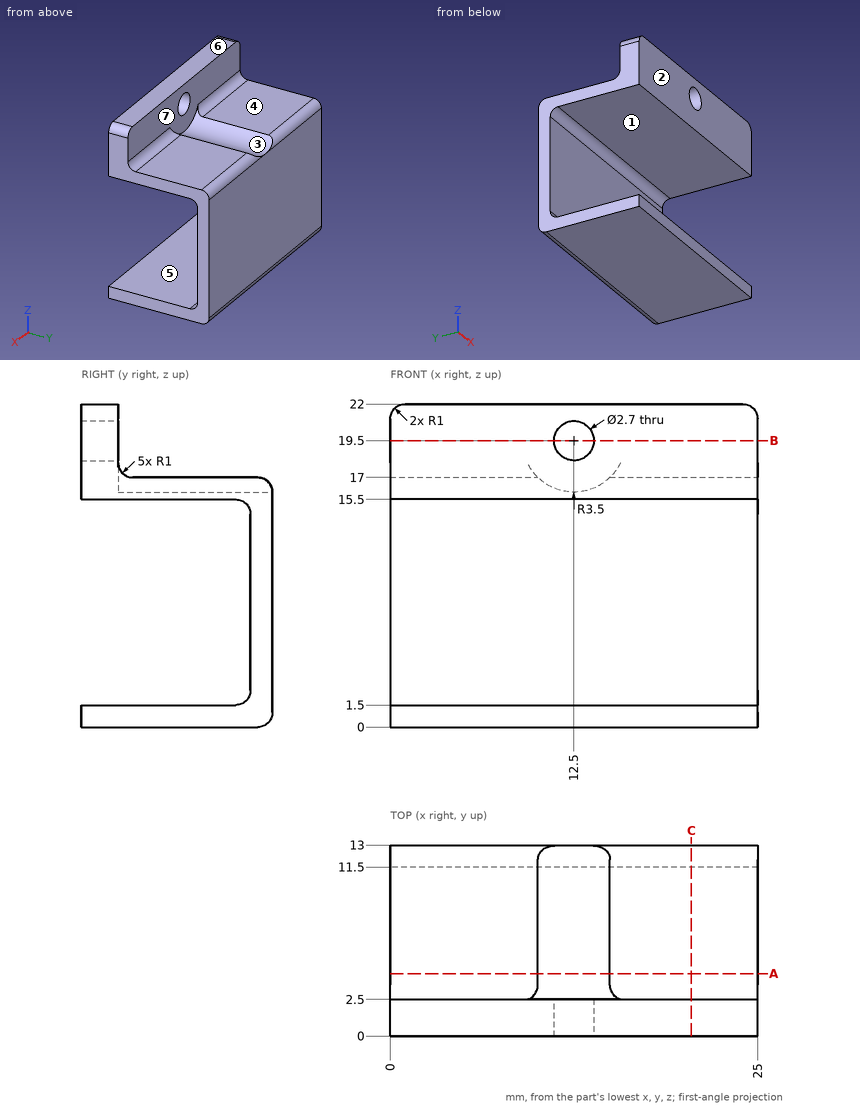
Check sheet for the drawn part. Datum: minimum x, y, z corner. Units: mm. A direction names the side the tool comes from. Round coordinates to 2 decimals unless told otherwise and drop trailing zeros. Order: outer loops, then holes, each group sorted by start corner. A loop starts at its lowest first (then second) coordinate and runs counter-clockwise, first axis right, second up. Notation, with made-up numbers: (4.25, 23) -> (38.25, 23) arc R22 cw to (38.25, 40) -> close; hole circle Ø9 at (23.25, -16). An arc over 180 degrees is marked (long way). Put each result on its own line as item: value. Start each with the question number.
(1) Depth check by flat-ended pin: pin 1 Ø5 at (x, y) = (6.5, 11.5) entering from +Z; pin 2 Ø2 at (x, z) = (10, 12) entering from -Y. Enter the tip coordinate at first touch or a pass-through.
(2) Section check C-C (x = 20.5). Enter the section's corners in (y, z).
(3) Tool access check on the marked faces 1, 2, 3 and 4. Record the directions out of +Z, -Z, +X, -X, +Y, -Y that give a thin tool (end or side, any length) a straight path to the whole face; none if there is none.
(4) Draft check along Z on the marked faces 5, 6 and 7. Enter one of: +Z half, -Z half, draft (parallel to the pull), parting line (faces both ways), or undercut.
(5) Material ranges on line 1 along Z through (x, y) = (12.5, 1.3); line 2 along Z through (x, y) = (17.25, 8.5); line 3 along X through (y, z) = (1.35, 19.5), recorded low to high.
(6) Section check A-A (y = 4.25). Enter the section's corners in (x, z).
(7) Section check B-B (z = 19.5). Enter the section's corners in (x, y).
Completed:
1. pin 1: stops at z = 17
1. pin 2: stops at y = 11.5
2. outline: (0, 0) -> (12, 0) arc R1 ccw to (13, 1) -> (13, 16) arc R1 ccw to (12, 17) -> (3.5, 17) arc R1 cw to (2.5, 18) -> (2.5, 22) -> (0, 22) -> (0, 15.5) -> (10.5, 15.5) arc R1 cw to (11.5, 14.5) -> (11.5, 2.5) arc R1 cw to (10.5, 1.5) -> (0, 1.5) -> close
3. face 1: +X, -X, -Y
3. face 2: +Z, -Z, +X, -X, -Y
3. face 3: +Z, +Y
3. face 4: +Z, +X, -X, +Y
4. face 5: undercut
4. face 6: +Z half
4. face 7: draft
5. line 1: z = 0 to 1.5, 15.5 to 18.15, 20.85 to 22
5. line 2: z = 0 to 1.5, 15.5 to 17
5. line 3: x = 0 to 11.15, 13.85 to 25
6. outline: (0, 0) -> (25, 0) -> (25, 1.5) -> (0, 1.5) -> close; (0, 15.5) -> (25, 15.5) -> (25, 17) -> (14.95, 17) arc R3.5 cw to (10.05, 17) -> (0, 17) -> close
7. outline: (0, 0) -> (11.15, 0) -> (11.15, 2.5) -> (0, 2.5) -> close; (13.85, 0) -> (25, 0) -> (25, 2.5) -> (13.85, 2.5) -> close
